```python
from build123d import *

# Parameters (mm, degrees)
SKETCH_1_W          = 100
SKETCH_1_H          = 100
EXTRUDE_1_DEPTH     = 840
SKETCH_2_W          = 92
SKETCH_2_H          = 92
CUT_EXTRUDE_1_DEPTH = 852.821577562
SKETCH_3_R          = 13
CUT_EXTRUDE_2_DEPTH = 852.821577562
CUT_EXTRUDE_3_DEPTH = 851.919502656


with BuildPart() as part:
    # 草图1 → 凸台-拉伸1 (new body)
    with BuildSketch(Plane.XY):
        with Locations((50, 50)):
            Rectangle(SKETCH_1_W, SKETCH_1_H)
    extrude(amount=EXTRUDE_1_DEPTH)

    # 草图2 → 切除-拉伸1 (cut, through all)
    with BuildSketch(Plane.XY.offset(840)):
        with Locations((54, 54)):
            Rectangle(SKETCH_2_W, SKETCH_2_H)
    extrude(amount=-CUT_EXTRUDE_1_DEPTH, mode=Mode.SUBTRACT)

    # 草图3 → 切除-拉伸2 (cut, through all)
    with BuildSketch(Plane.ZY):
        with Locations((43, 42)):
            Circle(SKETCH_3_R)
        with Locations((119, 66)):
            Circle(SKETCH_3_R)
        with Locations((797, 66)):
            Circle(SKETCH_3_R)
        with Locations((721, 42)):
            Circle(SKETCH_3_R)
    extrude(amount=-CUT_EXTRUDE_2_DEPTH, mode=Mode.SUBTRACT)

    # 草图4 → 切除-拉伸3 (cut, through all)
    with BuildSketch(Plane(origin=(0, 8, 0), x_dir=(1, 0, 0), z_dir=(0, 1, 0))):
        Polygon((15, 0), (15, -50), (100, -135), (100, 0), align=None)
        Polygon((15, -840), (15, -790), (100, -705), (100, -840), align=None)
    extrude(amount=-CUT_EXTRUDE_3_DEPTH, mode=Mode.SUBTRACT)


solid = part.part
```
Read the model definition and answer for the solid it produces. Units are mm, in the model's axes. A direction names the side the tool comes from. Coordinates: 2 decimals unless noted, no trailing zeros. Loops run counter-clockwise (first coordinate to the right, second up) from the corner with the lowest first, then second, coordinate; pieces in that order, holes last. Notation, with made-up numbers: (44, -30.5) - (55, -30.5) arc R21 ccw to (55, 1.5) - close; hole circle Ø10 at (68.5, 47.5). An arc over 180 degrees is marked (long way). Answer in a Markdown table with one row per item.
1. Straight lines are drawn through the part: line 1 (Y direction, x = 6, z = 119); line 2 (Y direction, x = 3.25, z = 721); line 3 (X direction, y = 23, z = 675). For each, find the intervals that lie inside material, in ascending order.
Conclusion:
| item | result |
|---|---|
| line 1 | y = 0 to 53, 79 to 100 |
| line 2 | y = 0 to 29, 55 to 100 |
| line 3 | x = 0 to 8 |
2. Find section D-D, the plane x = 67.5. Write down the section's boundary in (y, z).
Conclusion:
| item | result |
|---|---|
| outline | (0, 102.5) - (8, 102.5) - (8, 737.5) - (0, 737.5) - close |
3. Determine the mould class of faces 3 (the face through (3.9, 69.9, 131.4)), 4 (the face through (3.9, 45.9, 733.4)), 5 (the face through (49, 0, 414)), 6 (the face through (4, 51, 840)) for opening direction Z: +Z half, -Z half, draft (parallel to the pull), parting line (faces both ways), or undercut.
Conclusion:
| item | result |
|---|---|
| face 3 | undercut |
| face 4 | undercut |
| face 5 | draft |
| face 6 | +Z half |
4. Find section B-B, the plane y = 42. Write down the section's boundary in (x, z).
Conclusion:
| item | result |
|---|---|
| outline | (0, 0) - (8, 0) - (8, 30) - (0, 30) - close; (0, 56) - (8, 56) - (8, 708) - (0, 708) - close; (0, 734) - (8, 734) - (8, 840) - (0, 840) - close |
5. Find section C-C, the plane z = 291. Write down the section's boundary in (x, y), then the cut area to 3 significant figures.
Conclusion:
| item | result |
|---|---|
| outline | (0, 0) - (100, 0) - (100, 8) - (8, 8) - (8, 100) - (0, 100) - close |
| area | 1,540 mm² |
6. Given pin 1 (21 mm diameter, centred on y = 42, z = 43, fed in from +X); pin 2 (8 mm diameter, centred on x = 38.5, z = 732, fed in from +Y); pin 3 (1 mm diameter, centred on y = 29.5, z = 475.5, fed in from +X); pin 4 (9 mm diameter, centred on y = 3, z = 28.5, fed in from +X), each flat-ended and moving along its own axis, determine where each tip first touches the part or whether it passes through.
Conclusion:
| item | result |
|---|---|
| pin 1 | passes through |
| pin 2 | stops at y = 8 |
| pin 3 | stops at x = 8 |
| pin 4 | stops at x = 15 |
7. Find section A-A, the plane z = 721. Write down the section's boundary in (x, y).
Conclusion:
| item | result |
|---|---|
| outline | (0, 0) - (84, 0) - (84, 8) - (8, 8) - (8, 29) - (0, 29) - close; (0, 55) - (8, 55) - (8, 100) - (0, 100) - close |
8. Which of the six approach directions +Z, -Z, +X, -X, +Y, -Y give full straight-line access (tool end or side, diameter ignored) to faces 1 (the face through (53, 8, 426)), 2 (the face through (4, 51, 0))?
Conclusion:
| item | result |
|---|---|
| face 1 | +Z, -Z, +X, +Y |
| face 2 | -Z, +X, -X, +Y, -Y |
